from build123d import *

# Parameters (mm, degrees)
EXTRUDE1_DEPTH     = 60
CUT_EXTRUDE1_DEPTH = 53


with BuildPart() as part:
    # Sketch1 → Extrude1 (new body)
    with BuildSketch(Plane(origin=(0, 0, 0), x_dir=(1, 0, 0), z_dir=(0, 1, 0))):
        with BuildLine():
            Line((0, 40), (0, 52))
            Line((0, 52), (80, 52))
            Line((80, 52), (80, 18))
            Line((80, 18), (50, 0))
            Line((50, 0), (30, 10))
            ThreePointArc((30, 10), (21.213203436, 31.213203436), (0, 40))
        make_face()
    extrude(amount=EXTRUDE1_DEPTH)

    # Sketch2 → Cut-Extrude1 (cut, through all)
    with BuildSketch(Plane.XY):
        Polygon((0, 60), (0, 15), (50, 60), align=None)
        Polygon((80, 40), (80, 60), (50, 60), align=None)
    extrude(amount=-CUT_EXTRUDE1_DEPTH, mode=Mode.SUBTRACT)


solid = part.part
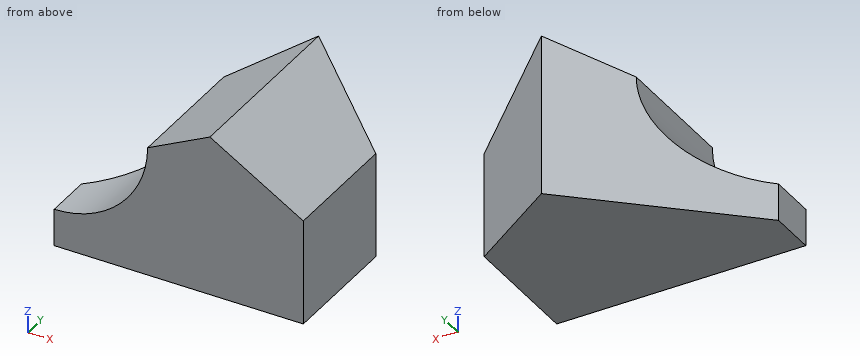
Check sheet for the modelled part. Datum: model origin and axes. Units: mm. Round coordinates to 2 decimals unless told otherwise and drop trailing zeros. Write each loop counter-clockwise with the first axis right and the second up, starting at its lowest first coordinate (ties: lowest second). Pieces come first, ordered by that corner, then holes. Notation, with made-up numbers: (-17.5, 18) - (1.5, 18) arc R9 ccw to (1.5, 24) - close; hole circle Ø6 at (26.25, 11). An arc over 180 degrees is marked (long way). Return JSON: item names as keys, results as strings.
Q1. Cross-section at D-D (z = -11.5). Record the boundary of the cut face in (x, y), then the cut area to 3 significant figures.
Returned:
{"outline": "(29.96, 0) - (69.17, 0) - (69.17, 47.22) - (50, 60) - (29.96, 41.97) - close", "area": "2,050 mm²"}
Q2. Scan lines: L1, parallel to Y at x = 37, z = -34.5; L2, parallel to Z at x = 41.5, y = 34; L3, parallel to Y at x = 52.5, z = -46.5. Record each from-to range of solid material in increasing order. Write a range as from..to.
Returned:
{"L1": "y = 0..48.3", "L2": "z = -52..-4.25", "L3": "y = 0..58.33"}
Q3. Cross-section at C-C (y = 36). Record the boundary of the cut face in (x, z).
Returned:
{"outline": "(23.33, -52) - (80, -52) - (80, -18) - (50, 0) - (30, -10) arc R30 cw to (23.33, -28.86) - close"}
Q4. Cross-section at A-A (z = -34). Record the boundary of the cut face in (x, y), then the cut area to 3 significant figures.
Returned:
{"outline": "(18, 0) - (80, 0) - (80, 40) - (50, 60) - (18, 31.2) - close", "area": "2,960 mm²"}
Q5. Depth check by flat-ended pin: P1, Ø8, axis at x = 59.5, y = 41.5, coming from the +Z side; P2, Ø10, axis at y = 18, z = -11.5, coming from the +X side; P3, Ø6, axis at y = 53, z = -40, coming from the +X side. Enter the tip coordinate at first touch or a pass-through.
Returned:
{"P1": "stops at z = -3.3", "P2": "stops at x = 77.5", "P3": "stops at x = 65"}
Q6. Cross-section at B-B (x = 45). Record the boundary of the cut face in (y, z), then the cut area to 3 significant figures.
Returned:
{"outline": "(0, -52) - (55.5, -52) - (55.5, -2.5) - (0, -2.5) - close", "area": "2,750 mm²"}
